The model under review builds one solid part; all positions refer to its coordinate system, in mm. Face numbers are marked on the shaded views. Round coordinates to 2 decimals unless told otherwise and drop trailing zeros. Write each loop counter-clockwise with the first axis right and the second up, starting at its lowest first coordinate (ties: lowest second). Pieces come first, ordered by that corner, then holes. Notation, with made-up numbers: (48, 57) -> (105, 57) arc R13 cw to (105, 74) -> close; hole circle Ø7 at (-6.75, -8.5). An arc over 180 degrees is marked (long way). Use CSV: the item, a comma, the result in double quotes. Start each with the question number.
1) Mouldability with a two-part tool opening along X and no side actions: class the marked faces 1, 2, 3 and 4 as released by +X, released by -X, zero draft, split by the parting line, or undercut.
2) Take a section at C-C, the plane z = 2. Give the boundary of the cut face in (x, y) (3 decimals), then the cut area to 3 significant figures.
3) Take a section at D-D, the plane z = 8. Give the boundary of the cut face in (x, y) (3 decimals).
4) Take a section at B-B, the plane y = 1.5. Give the boundary of the cut face in (x, z) (3 decimals).
5) For pin 1 Ø5.5 at (x, z) = (15.24, 1.27) entering from -Y, flat-tipped, find the tip position at first contact; note if it passes through.
6) Take a section at A-A, the plane x = 10.75. Give the boundary of the cut face in (y, z) (3 decimals).
7) Wall thickness on probe 1 along Z at (x, y) = (15.24, 0.85); probe 2 along Z at (x, y) = (13.75, 2.1); probe 3 along X at (y, z) = (0.7, 8.25): over which ranges is each line inside the solid? List them lowest first. Write a range as [from, to].
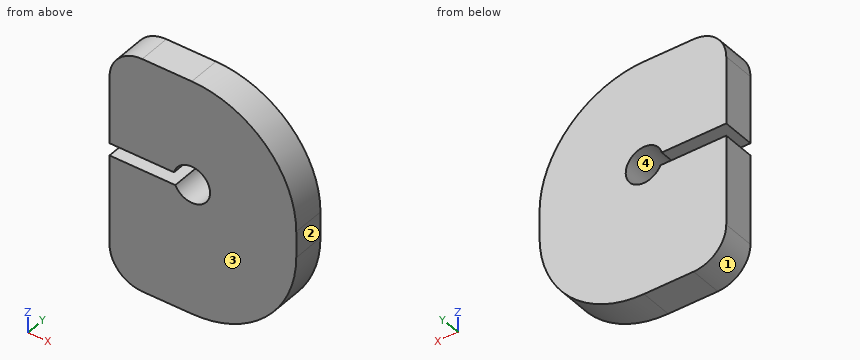
from build123d import *

# Parameters (mm, degrees)
SKETCH1_W           = 50.8
SKETCH1_H           = 22.86
BOSS_EXTRUDE1_DEPTH = 3.175
FILLET1_R           = 10.16
SKETCH3_R           = 1.778
CUT_EXTRUDE1_DEPTH  = 29.033649869
FILLET3_R           = 10.16
SKETCH4_W           = 32.639
SKETCH4_H           = 22.86
CUT_EXTRUDE2_DEPTH  = 29.033649869
FILLET9_R           = 3.175
SKETCH5_W           = 6.800031064
SKETCH5_H           = 1.2
CUT_EXTRUDE4_DEPTH  = 29.033649869


with BuildPart() as part:
    # Sketch1 → Boss-Extrude1 (new body)
    with BuildSketch(Plane(origin=(0, 0, 0), x_dir=(1, 0, 0), z_dir=(0, 1, 0))):
        Rectangle(SKETCH1_W, SKETCH1_H)
    extrude(amount=BOSS_EXTRUDE1_DEPTH)

    # Fillet1
    fillet1_edges = [part.edges().sort_by_distance(p)[0] for p in [
        (25.4, 1.5875, 11.43),
        (-25.4, 1.5875, 11.43),
    ]]
    fillet(fillet1_edges, radius=FILLET1_R)

    # Sketch3 → Cut-Extrude1 (cut, through all)
    with BuildSketch(Plane(origin=(0, 3.175, 0), x_dir=(1, 0, 0), z_dir=(0, 1, 0))):
        with Locations(Location((15.24, -1.27, 0), (0, 0, 270))):
            Circle(SKETCH3_R)
        with Locations(Location((-3.81, -1.27, 0), (0, 0, 270))):
            Circle(SKETCH3_R)
    extrude(amount=-CUT_EXTRUDE1_DEPTH, mode=Mode.SUBTRACT)

    # Fillet3
    fillet3_edges = [part.edges().sort_by_distance(p)[0] for p in [
        (-25.4, 1.5875, -11.43),
        (25.4, 1.5875, -11.43),
    ]]
    fillet(fillet3_edges, radius=FILLET3_R)

    # Sketch4 → Cut-Extrude2 (cut, through all)
    with BuildSketch(Plane(origin=(0, 3.175, 0), x_dir=(1, 0, 0), z_dir=(0, 1, 0))):
        with Locations((-9.0805, 0)):
            Rectangle(SKETCH4_W, SKETCH4_H)
    extrude(amount=-CUT_EXTRUDE2_DEPTH, mode=Mode.SUBTRACT)

    # Fillet9
    fillet9_edges = [part.edges().sort_by_distance(p)[0] for p in [
        (7.239, 1.5875, -11.43),
        (7.239, 1.5875, 11.43),
    ]]
    fillet(fillet9_edges, radius=FILLET9_R)

    # Sketch5 → Cut-Extrude4 (cut, through all)
    with BuildSketch(Plane(origin=(0, 3.175, 0), x_dir=(1, 0, 0), z_dir=(0, 1, 0))):
        with Locations((10.639015532, -1.100889409)):
            Rectangle(SKETCH5_W, SKETCH5_H)
    extrude(amount=-CUT_EXTRUDE4_DEPTH, mode=Mode.SUBTRACT)


solid = part.part
Values found:
1,face 1,"released by -X"
1,face 2,"released by +X"
1,face 3,"zero draft"
1,face 4,"undercut"
2,outline,"(7.239, 0) -> (13.619, 0) -> (13.619, 3.175) -> (7.239, 3.175) -> close; (16.861, 0) -> (25.374, 0) -> (25.374, 3.175) -> (16.861, 3.175) -> close"
2,area,"47.3 mm²"
3,outline,"(7.239, 0) -> (22.851, 0) -> (22.851, 3.175) -> (7.239, 3.175) -> close"
4,outline,"(7.239, -8.255) arc R3.175 ccw to (10.414, -11.43) -> (15.24, -11.43) arc R10.16 ccw to (25.4, -1.27) -> (25.4, 1.27) arc R10.16 ccw to (15.24, 11.43) -> (10.414, 11.43) arc R3.175 ccw to (7.239, 8.255) -> (7.239, 1.701) -> (13.515, 1.701) arc R1.778 cw (long way) to (13.637, 0.501) -> (7.239, 0.501) -> close"
5,pin 1,"y = 0"
6,outline,"(0, -11.43) -> (3.175, -11.43) -> (3.175, 0.501) -> (0, 0.501) -> close; (0, 1.701) -> (3.175, 1.701) -> (3.175, 11.43) -> (0, 11.43) -> close"
7,probe 1,"[-11.43, -0.51], [3.05, 11.43]"
7,probe 2,"[-11.43, 0.3], [2.24, 11.43]"
7,probe 3,"[7.24, 22.62]"
